from build123d import *

# Parameters (mm, degrees)
SKETCH_1_W                      = 40
SKETCH_1_H                      = 50
SKETCH_1_W_2                    = 35
SKETCH_1_H_2                    = 43.75
EXTRUDE_1_DEPTH                 = 20
CHAMFER_1_SIZE                  = 2
SKETCH_4_R                      = 1.5
CUT_EXTRUDE_3_DEPTH             = 6
SKETCH_7_W                      = 8
SKETCH_7_H                      = 46
EXTRUDE_2_DEPTH                 = 26
SKETCH_8_W                      = 8
SKETCH_8_H                      = 26
CUT_EXTRUDE_5_DEPTH             = 12
CHAMFER_2_SIZE                  = 2
FILLET_1_R                      = 4
CUT_EXTRUDE_6_DEPTH             = 70.426219831
CUT_EXTRUDE_6_DEPTH_BACK        = 70.426219831
SKETCH_9_R                      = 1.5
SKETCH_10_W                     = 35
SKETCH_10_H                     = 43.75
EXTRUDE_4_DEPTH                 = 2
SKETCH_11_W                     = 62
SKETCH_11_H                     = 100
SKETCH_11_R                     = 1.4
SKETCH_11_W_2                   = 35
SKETCH_11_H_2                   = 43.75
EXTRUDE_5_DEPTH                 = 3
FILLET_2_R                      = 5
SKETCH_12_W                     = 35
SKETCH_12_H                     = 43.75
EXTRUDE_6_DEPTH                 = 11
CUT_EXTRUDE_4_REACH             = 92.94
SKETCH_5_R                      = 1.5
CUT_EXTRUDE_4_DIRECTION_2_DEPTH = 91.939540355


with BuildPart() as part:
    # 草图1 → 凸台-拉伸1 (new body)
    with BuildSketch(Plane.XY):
        Rectangle(SKETCH_1_W, SKETCH_1_H)
        Rectangle(SKETCH_1_W_2, SKETCH_1_H_2, mode=Mode.SUBTRACT)
    extrude(amount=EXTRUDE_1_DEPTH)

    # 倒角1
    chamfer_1_edges = [part.edges().sort_by_distance(p)[0] for p in [
        (20, -25, 10),
        (-20, -25, 10),
        (-20, 25, 10),
        (20, 25, 10),
    ]]
    chamfer(chamfer_1_edges, length=CHAMFER_1_SIZE)

    # 草图4 → 切除-拉伸3 (cut)
    with BuildSketch(Plane(origin=(0, 25, 0), x_dir=(1, 0, 0), z_dir=(0, 1, 0))):
        with Locations(Location((-12, -4, 0), (0, 0, 270))):
            Circle(SKETCH_4_R)
        with Locations(Location((0, -4, 0), (0, 0, 270))):
            Circle(SKETCH_4_R)
        with Locations(Location((12, -4, 0), (0, 0, 270))):
            Circle(SKETCH_4_R)
    extrude(amount=-CUT_EXTRUDE_3_DEPTH, mode=Mode.SUBTRACT)

    # 草图7 → 凸台-拉伸2 (add)
    with BuildSketch(Plane(origin=(20, 0, 0), x_dir=(0, 0, -1), z_dir=(1, 0, 0))):
        with Locations((-16, 0)):
            Rectangle(SKETCH_7_W, SKETCH_7_H)
    extrude(amount=EXTRUDE_2_DEPTH)

    # 草图8 → 切除-拉伸5 (cut)
    with BuildSketch(Plane(origin=(46, 0, 0), x_dir=(0, 0, -1), z_dir=(1, 0, 0))):
        with Locations((-16, 0)):
            Rectangle(SKETCH_8_W, SKETCH_8_H)
    extrude(amount=-CUT_EXTRUDE_5_DEPTH, mode=Mode.SUBTRACT)

    # 倒角2
    chamfer_2_edges = [part.edges().sort_by_distance(p)[0] for p in [
        (46, -23, 16),
        (46, 23, 16),
    ]]
    chamfer(chamfer_2_edges, length=CHAMFER_2_SIZE)

    # 圆角1
    fillet_1_edges = [part.edges().sort_by_distance(p)[0] for p in [
        (46, -17, 12),
        (46, -17, 20),
        (46, 17, 12),
        (46, 17, 20),
    ]]
    fillet(fillet_1_edges, radius=FILLET_1_R - 0.0001)  # a hair under: the kernel refuses the full size

    # 草图9 → 切除-拉伸6 (cut, two sides: drawn at the far end of the back side and taken through both)
    with BuildSketch(Plane.XZ.offset(23).offset(-CUT_EXTRUDE_6_DEPTH_BACK)):
        with Locations((40, 16)):
            Circle(SKETCH_9_R)
    extrude(amount=CUT_EXTRUDE_6_DEPTH + CUT_EXTRUDE_6_DEPTH_BACK, mode=Mode.SUBTRACT)

    # 草图10 → 凸台-拉伸4 (add)
    with BuildSketch(Plane(origin=(0, 0, 0), x_dir=(-1, 0, 0), z_dir=(0, 0, -1))):
        Rectangle(SKETCH_10_W, SKETCH_10_H)
    extrude(amount=-EXTRUDE_4_DEPTH)

    # 草图11 → 凸台-拉伸5 (add)
    with BuildSketch(Plane.XY.offset(20)):
        with Locations((-11, 0)):
            Rectangle(SKETCH_11_W, SKETCH_11_H)
        with Locations((-38, 46)):
            Circle(SKETCH_11_R, mode=Mode.SUBTRACT)
        with Locations((16, 46)):
            Circle(SKETCH_11_R, mode=Mode.SUBTRACT)
        with Locations((-38, -46)):
            Circle(SKETCH_11_R, mode=Mode.SUBTRACT)
        with Locations((16, -46)):
            Circle(SKETCH_11_R, mode=Mode.SUBTRACT)
        Rectangle(SKETCH_11_W_2, SKETCH_11_H_2, mode=Mode.SUBTRACT)
    extrude(amount=EXTRUDE_5_DEPTH)

    # 圆角2
    fillet_2_edges = [part.edges().sort_by_distance(p)[0] for p in [
        (20, -50, 21.5),
        (20, 50, 21.5),
        (-42, 50, 21.5),
        (-42, -50, 21.5),
    ]]
    fillet(fillet_2_edges, radius=FILLET_2_R)

    # 草图12 → 凸台-拉伸6 (add)
    with BuildSketch(Plane.XY.offset(2)):
        Rectangle(SKETCH_12_W, SKETCH_12_H)
    extrude(amount=EXTRUDE_6_DEPTH)

    # 草图5 → 切除-拉伸4 (cut, up to next)
    with BuildSketch(Plane.XZ.offset(25), mode=Mode.PRIVATE) as cut_extrude_4_sk1:
        with Locations(Location((-12, 4, 0), (0, 0, 90))):
            Circle(SKETCH_5_R)
    cut_extrude_4_tool1 = extrude(cut_extrude_4_sk1.sketch, amount=-CUT_EXTRUDE_4_REACH, mode=Mode.PRIVATE) & part.part
    # 草图5 → 切除-拉伸4 (cut, up to next)
    with BuildSketch(Plane.XZ.offset(25), mode=Mode.PRIVATE) as cut_extrude_4_sk2:
        with Locations(Location((0, 4, 0), (0, 0, 90))):
            Circle(SKETCH_5_R)
    cut_extrude_4_tool2 = extrude(cut_extrude_4_sk2.sketch, amount=-CUT_EXTRUDE_4_REACH, mode=Mode.PRIVATE) & part.part
    # 草图5 → 切除-拉伸4 (cut, up to next)
    with BuildSketch(Plane.XZ.offset(25), mode=Mode.PRIVATE) as cut_extrude_4_sk3:
        with Locations(Location((12, 4, 0), (0, 0, 90))):
            Circle(SKETCH_5_R)
    cut_extrude_4_tool3 = extrude(cut_extrude_4_sk3.sketch, amount=-CUT_EXTRUDE_4_REACH, mode=Mode.PRIVATE) & part.part
    add(cut_extrude_4_tool1.solids().sort_by_distance((-12, -25, 4))[0], mode=Mode.SUBTRACT)
    add(cut_extrude_4_tool2.solids().sort_by_distance((0, -25, 4))[0], mode=Mode.SUBTRACT)
    add(cut_extrude_4_tool3.solids().sort_by_distance((12, -25, 4))[0], mode=Mode.SUBTRACT)

    # 草图5 → 切除-拉伸4 direction 2 (cut)
    with BuildSketch(Plane.XZ.offset(25)):
        with Locations(Location((-12, 4, 0), (0, 0, 90))):
            Circle(SKETCH_5_R)
        with Locations(Location((0, 4, 0), (0, 0, 90))):
            Circle(SKETCH_5_R)
        with Locations(Location((12, 4, 0), (0, 0, 90))):
            Circle(SKETCH_5_R)
    extrude(amount=CUT_EXTRUDE_4_DIRECTION_2_DEPTH, mode=Mode.SUBTRACT)


solid = part.part
Part model, mm, in its own coordinate system. A direction names the side the tool comes from. Coordinates: 2 decimals unless noted, no trailing zeros. Order: outer loops, then holes, each group sorted by start corner. A loop starts at its lowest first (then second) coordinate and runs counter-clockwise, first axis right, second up.
(1) Slice it at C-C, the plane y = -17. State how many separate pieces and enclosed holes the cut face has, and give its area (3 significant figures).
Check sheet entries:
separate pieces: 1
enclosed holes: 4
area: 809 mm2
(2) Slice it at D-D, the plane z = 10.5. Write the cut outline in (x, y), and give its area (3 significant figures).
Check sheet entries:
outline: (-20, -23) - (-18, -25) - (18, -25) - (20, -23) - (20, 23) - (18, 25) - (-18, 25) - (-20, 23) - close
area: 1,990 mm2
(3) Probe L1, parallel to X at y = 3, z = 4; L2, parallel to X at y = -16, z = 20.25; L3, parallel to Y at x = -38, z = 21.5. List the from-to ranges inside material, lowest first.
Check sheet entries:
L1: x = -20 to -13.5, -10.5 to -1.5, 1.5 to 10.5, 13.5 to 20
L2: x = -42 to -17.5, 17.5 to 20
L3: y = -49.9 to -47.4, -44.6 to 44.6, 47.4 to 49.9
(4) Pull direction Y, two halves, no side cores. Call faces 1 (the face through (-17.5, 0, 18)), 2 (the face through (-41, 48, 22)), 3 (the face through (-11, -50, 21)): pulls with the +Y half, pulls with the -Y half, needs draft (parallel to the pull), parting line crosses it, or undercut.
Check sheet entries:
face 1: undercut
face 2: pulls with the +Y half
face 3: pulls with the -Y half
(5) Slice it at A-A, the plane x = 0. Write the cut outline in (y, z) (3 decimals).
Check sheet entries:
outline: (-50, 20) - (-25, 20) - (-25, 5.5) - (25, 5.5) - (25, 20) - (50, 20) - (50, 23) - (21.875, 23) - (21.875, 13) - (-21.875, 13) - (-21.875, 23) - (-50, 23) - close; (-25, 0) - (25, 0) - (25, 2.5) - (-25, 2.5) - close
(6) Slice it at B-B, the plane z = 4. Write the cut outline in (x, y).
Check sheet entries:
outline: (-20, -23) - (-18, -25) - (-13.5, -25) - (-13.5, 25) - (-18, 25) - (-20, 23) - close; (-10.5, -25) - (-1.5, -25) - (-1.5, 25) - (-10.5, 25) - close; (1.5, -25) - (10.5, -25) - (10.5, 25) - (1.5, 25) - close; (13.5, -25) - (18, -25) - (20, -23) - (20, 23) - (18, 25) - (13.5, 25) - close
(7) Pin check, flat tips, straight feed: pin 1 Ø8 at (x, z) = (21, 2.5) entering from -Y; pin 2 Ø1.5 at (y, z) = (-10.5, 21) entering from +X; pin 3 Ø6 at (x, z) = (24.5, 13) entering from +Y. Stop position of each tip, or through.
Check sheet entries:
pin 1: stops at y = -25
pin 2: stops at x = 20
pin 3: stops at y = 23
(8) Tool access for faces 4 (the face through (32, 23, 16)), 5 (the face through (0, 25, 10)), 6 (the face through (0, -25, 10)): list every direction of +Z, -Z, +X, -X, +Y, -Y with a clear straight run to the whole face (end or side of a thin tool).
Check sheet entries:
face 4: +Z, -Z, +X, +Y
face 5: -Z, +X, -X, +Y
face 6: -Z, +X, -X, -Y
